from build123d import *

# Parameters (mm, degrees)
SKETCH1_W           = 35
SKETCH1_H           = 30
BOSS_EXTRUDE1_DEPTH = 1.5
SKETCH2_R           = 1.65
CUT_EXTRUDE1_DEPTH  = 3
SKETCH3_W           = 20
SKETCH3_H           = 30
BOSS_EXTRUDE2_DEPTH = 40
SKETCH4_W           = 30
SKETCH4_H           = 18
BOSS_EXTRUDE3_DEPTH = 2.5
CUT_EXTRUDE2_DEPTH  = 30
SKETCH7_R           = 1.65
CUT_EXTRUDE3_DEPTH  = 25


with BuildPart() as part:
    # Sketch1 → Boss-Extrude1 (new body, symmetric)
    with BuildSketch(Plane(origin=(0, 0, 0), x_dir=(1, 0, 0), z_dir=(0, 1, 0))):
        Rectangle(SKETCH1_W, SKETCH1_H)
    extrude(amount=BOSS_EXTRUDE1_DEPTH, both=True)

    # Sketch2 → Cut-Extrude1 (cut)
    with BuildSketch(Plane(origin=(0, 1.5, 0), x_dir=(1, 0, 0), z_dir=(0, 1, 0))):
        with Locations((-13.5, 11)):
            Circle(SKETCH2_R)
        with Locations((13.5, 11)):
            Circle(SKETCH2_R)
        with Locations((13.5, -11)):
            Circle(SKETCH2_R)
        with Locations((-13.5, -11)):
            Circle(SKETCH2_R)
    extrude(amount=-CUT_EXTRUDE1_DEPTH, mode=Mode.SUBTRACT)

    # Sketch3 → Boss-Extrude2 (add)
    with BuildSketch(Plane(origin=(0, 1.5, 0), x_dir=(1, 0, 0), z_dir=(0, 1, 0))):
        Rectangle(SKETCH3_W, SKETCH3_H)
    extrude(amount=BOSS_EXTRUDE2_DEPTH)

    # Sketch4 → Boss-Extrude3 (add)
    with BuildSketch(Plane(origin=(10, 0, 0), x_dir=(0, 0, -1), z_dir=(1, 0, 0))):
        with Locations((0, 32.5)):
            Rectangle(SKETCH4_W, SKETCH4_H)
    boss_extrude3 = extrude(amount=BOSS_EXTRUDE3_DEPTH)

    # Mirror1: Boss-Extrude3 across plane
    add(boss_extrude3.mirror(Plane(origin=(0, 0, 0), x_dir=(0, 0, 1), z_dir=(1, 0, 0))))

    # Sketch5 → Cut-Extrude2 (cut)
    with BuildSketch(Plane(origin=(0, 0, -15), x_dir=(-1, 0, 0), z_dir=(0, 0, -1))):
        Polygon((0, 25.439594924), (5.377813855, 38.5), (-5.377813855, 38.5), align=None)
        Polygon((7, 8.439594924), (7, 34.560405076), (1.622186145, 21.5), align=None)
        Polygon((-7, 8.439594924), (-1.622186145, 21.5), (-7, 34.560405076), align=None)
        Polygon((5.377813855, 4.5), (0, 17.560405076), (-5.377813855, 4.5), align=None)
    extrude(amount=-CUT_EXTRUDE2_DEPTH, mode=Mode.SUBTRACT)

    # Sketch7 → Cut-Extrude3 (cut)
    with BuildSketch(Plane.ZY.offset(12.5)):
        with Locations((0, 37.5)):
            Circle(SKETCH7_R)
        with Locations((0, 29.5)):
            Circle(SKETCH7_R)
    extrude(amount=-CUT_EXTRUDE3_DEPTH, mode=Mode.SUBTRACT)


solid = part.part
Work out the finished part from the listing and answer in its coordinate system (mm). A direction names the side the tool comes from. Coordinates: 2 decimals unless noted, no trailing zeros. Loops run counter-clockwise (first coordinate to the right, second up) from the corner with the lowest first, then second, coordinate; pieces in that order, holes last. Notation, with made-up numbers: (19, 68.25) -> (60, 68.25) arc R15 cw to (60, 88.25) -> close; hole circle Ø11 at (80.25, 36.5). An arc over 180 degrees is marked (long way). Write each question's results on one line, items separated by ' | '. Start each with the question number.
1) Find section A-A on x = -13.5. Determine the outline of the cut face in (y, z), then the cut area to 3 significant figures.
2) Flat-ended cylindrical pins translate along their axes: P1, Ø4.5, axis at y = 29.5, z = 0, coming from the +X side; P2, Ø5, axis at y = 25.5, z = -10.5, coming from the -X side; P3, Ø11, axis at y = 11, z = -1, coming from the +X side; P4, Ø2.5, axis at x = -13.5, z = 11, coming from the +Y side. Find the tip coordinate at first contact, or state that the pin passes through.
3) Find section D-D on y = 14. Determine the outline of the cut face in (x, z), then the cut area to 3 significant figures.
4) Find section B-B on z = 7. Determine the outline of the cut face in (x, y), then the cut area to 3 significant figures.
5) For faces 4 (the flat face through (0, 38.5, -8)), 5 (the flat face through (12.5, 33, 0)), 6 (the cylindrical face through (15.024, 0.021, 11.632)), determine the directions among +Z, -Z, +X, -X, +Y, -Y from which every point of the face is accessible in a straight line to the end or side of a thin tool.
6) The mould has two halves that part along Z. Classify faces 1 (the flat face through (0, 20, -15)), 2 (the cylindrical face through (-3.33, 28.5, -1.31)), 3 (the flat face through (2.65, 11.12, -0.21)): pulls with the +Z half, pulls with the -Z half, needs draft (parallel to the pull), parting line crosses it, or undercut.
7) Find section C-C on y = 34. Determine the outline of the cut face in (x, z), then the cut area to 3 significant figures.
8) Consider line 1 along Y through (x, z) = (9.65, 0); line 2 along X through (y, z) = (12, -10); line 3 along X through (y, z) = (1, 10). Determine where each line is inside the solid, lowest interval first.
Response values:
1) outline: (-1.5, -15) -> (1.5, -15) -> (1.5, -12.65) -> (-1.5, -12.65) -> close; (-1.5, -9.35) -> (1.5, -9.35) -> (1.5, 9.35) -> (-1.5, 9.35) -> close; (-1.5, 12.65) -> (1.5, 12.65) -> (1.5, 15) -> (-1.5, 15) -> close | area: 70.2 mm^2
2) P1: stops at x = 12.5 | P2: stops at x = -12.5 | P3: stops at x = 10 | P4: stops at y = 41.5
3) outline: (-10, -15) -> (-7, -15) -> (-7, 15) -> (-10, 15) -> close; (-4.71, -15) -> (-1.47, -15) -> (-1.47, 15) -> (-4.71, 15) -> close; (1.47, -15) -> (4.71, -15) -> (4.71, 15) -> (1.47, 15) -> close; (7, -15) -> (10, -15) -> (10, 15) -> (7, 15) -> close | area: 375 mm^2
4) outline: (-17.5, -1.5) -> (17.5, -1.5) -> (17.5, 1.5) -> (10, 1.5) -> (10, 23.5) -> (12.5, 23.5) -> (12.5, 41.5) -> (-12.5, 41.5) -> (-12.5, 23.5) -> (-10, 23.5) -> (-10, 1.5) -> (-17.5, 1.5) -> close; hole (-7, 8.44) -> (-1.62, 21.5) -> (-7, 34.56) -> close; hole (-5.38, 4.5) -> (5.38, 4.5) -> (0, 17.56) -> close; hole (-5.38, 38.5) -> (0, 25.44) -> (5.38, 38.5) -> close; hole (1.62, 21.5) -> (7, 8.44) -> (7, 34.56) -> close | area: 714 mm^2
5) face 4: +Z, -Z | face 5: +Z, -Z, +X, +Y | face 6: -Y
6) face 1: pulls with the -Z half | face 2: undercut | face 3: needs draft
7) outline: (-12.5, -15) -> (-7, -15) -> (-7, 15) -> (-12.5, 15) -> close; (-6.77, -15) -> (-3.52, -15) -> (-3.52, 15) -> (-6.77, 15) -> close; (3.52, -15) -> (6.77, -15) -> (6.77, 15) -> (3.52, 15) -> close; (7, -15) -> (12.5, -15) -> (12.5, 15) -> (7, 15) -> close | area: 525 mm^2
8) line 1: y = -1.5 to 27.85, 31.15 to 35.85, 39.15 to 41.5 | line 2: x = -10 to -7, -5.53 to -2.29, 2.29 to 5.53, 7 to 10 | line 3: x = -17.5 to -14.81, -12.19 to 12.19, 14.81 to 17.5
